```python
from build123d import *

# Parameters (mm, degrees)
SKETCH2_R           = 3.65
BOSS_EXTRUDE1_DEPTH = 1.4
SKETCH3_R           = 2.8
BOSS_EXTRUDE2_DEPTH = 5.2
SKETCH4_R           = 3.65
BOSS_EXTRUDE3_DEPTH = 1.4
CUT_EXTRUDE1_DEPTH  = 9
CUT_EXTRUDE2_DEPTH  = 14.65


with BuildPart() as part:
    # Sketch2 → Boss-Extrude1 (new body)
    with BuildSketch(Plane(origin=(0, 0, 0), x_dir=(1, 0, 0), z_dir=(0, 1, 0))):
        Circle(SKETCH2_R)
    extrude(amount=BOSS_EXTRUDE1_DEPTH)

    # Sketch3 → Boss-Extrude2 (add)
    with BuildSketch(Plane(origin=(0, 1.4, 0), x_dir=(1, 0, 0), z_dir=(0, 1, 0))):
        Circle(SKETCH3_R)
    extrude(amount=BOSS_EXTRUDE2_DEPTH)

    # Sketch4 → Boss-Extrude3 (add)
    with BuildSketch(Plane(origin=(0, 6.6, 0), x_dir=(1, 0, 0), z_dir=(0, 1, 0))):
        Circle(SKETCH4_R)
    extrude(amount=BOSS_EXTRUDE3_DEPTH)

    # Sketch5 → Cut-Extrude1 (cut, through all)
    with BuildSketch(Plane(origin=(0, 8, 0), x_dir=(1, 0, 0), z_dir=(0, 1, 0))):
        Polygon((0.85, -2.351063589), (0.85, -0.85), (2.351063589, -0.85), (2.351063589, 0.85), (0.85, 0.85), (0.85, 2.351063589), (-0.85, 2.351063589), (-0.85, 0.85), (-2.351063589, 0.85), (-2.351063589, -0.85), (-0.85, -0.85), (-0.85, -2.351063589), align=None)
    extrude(amount=-CUT_EXTRUDE1_DEPTH, mode=Mode.SUBTRACT)

    # Sketch6 → Cut-Extrude2 (cut, through all)
    with BuildSketch(Plane(origin=(10, 0, 0), x_dir=(0, 0, -1), z_dir=(1, 0, 0))):
        with BuildLine():
            Line((0.5, 6.098665366), (0.5, 1.901334634))
            ThreePointArc((0.5, 1.901334634), (0, 1.401334634), (-0.5, 1.901334634))
            Line((-0.5, 1.901334634), (-0.5, 6.098665366))
            ThreePointArc((-0.5, 6.098665366), (0, 6.598665366), (0.5, 6.098665366))
        make_face()
    extrude(amount=-CUT_EXTRUDE2_DEPTH, mode=Mode.SUBTRACT)


solid = part.part
```
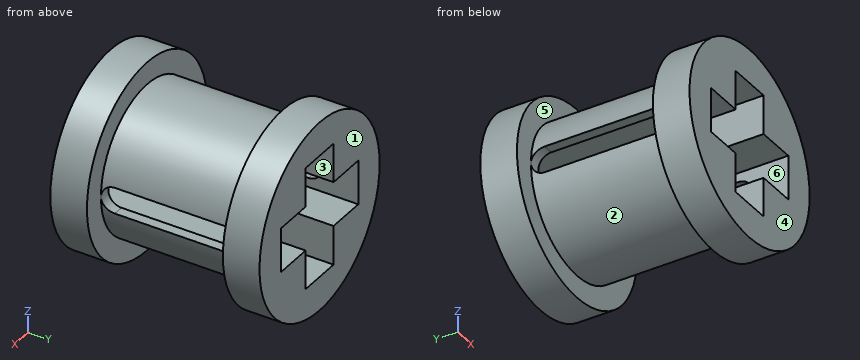
Part model, mm, in its own coordinate system. Face numbers are marked on the shaded views. A direction names the side the tool comes from. Round coordinates to 2 decimals unless told otherwise and drop trailing zeros. Loops run counter-clockwise (first coordinate to the right, second up) from the corner with the lowest first, then second, coordinate; pieces in that order, holes last.
Item 1: Drill centre lines: line 1 (Y direction, x = 0, z = 3); line 2 (X direction, y = 0.75, z = 1.5); line 3 (X direction, y = 2.5, z = -2). Where is each one in solid material? Low to high.
Item 2: Cut at D-D, the plane z = 1. Give the cut face in (x, y), then the cut area to 3 significant figures.
Item 3: Cut at A-A, the plane x = 0. Give the cut face in (y, z), then the cut area to 3 significant figures.
Item 4: Drop flat-ended pins along their axis: P1, Ø1.2, axis at y = 4, z = 2, coming from the +X side; P2, Ø2, axis at y = 6.5, z = 2, coming from the +X side; P3, Ø1.7, axis at x = 2, y = 3, coming from the +Z side. Give the stop position or say it passes through.
Item 5: Cut at B-B, the plane z = 0. State how many separate pieces and enclosed holes the cut face has, then the cut area to 3 significant figures.
Item 6: Mould opens along Z. For the marked faces 1, 2 and 3 say: +Z half, -Z half, draft (parallel to the pull), parting line (faces both ways), or undercut.
Item 7: 3-axis set-ups, long thin cutter, end or side, ignore diameter. For the marked faces 4, 5 and 6: which of +Z, -Z, +X, -X, +Y, -Y reach the whole face in a straight line?
Item 8: Cut at C-C, the plane y = 0.5. Give the cut face in (x, z).
A:
1. line 1: y = 0 to 1.4, 6.6 to 8
1. line 2: x = -3.33 to -0.85, 0.85 to 3.33
1. line 3: x = -1.96 to -0.85, 0.85 to 1.96
2. outline: (-3.51, 0) - (-0.85, 0) - (-0.85, 8) - (-3.51, 8) - (-3.51, 6.6) - (-2.62, 6.6) - (-2.62, 1.4) - (-3.51, 1.4) - close; (0.85, 0) - (3.51, 0) - (3.51, 1.4) - (2.62, 1.4) - (2.62, 6.6) - (3.51, 6.6) - (3.51, 8) - (0.85, 8) - close
2. area: 33.3 mm2
3. outline: (0, -3.65) - (1.4, -3.65) - (1.4, -2.8) - (6.6, -2.8) - (6.6, -3.65) - (8, -3.65) - (8, -2.35) - (0, -2.35) - close; (0, 2.35) - (8, 2.35) - (8, 3.65) - (6.6, 3.65) - (6.6, 2.8) - (1.4, 2.8) - (1.4, 3.65) - (0, 3.65) - close
3. area: 11.9 mm2
4. P1: stops at x = 2.42
4. P2: stops at x = 3.51
4. P3: stops at z = 2.55
5. separate pieces: 4
5. enclosed holes: 0
5. area: 7.28 mm2
6. face 1: draft
6. face 2: parting line
6. face 3: undercut
7. face 4: +Z, -Z, +X, -X, -Y
7. face 5: none
7. face 6: +Y, -Y
8. outline: circle Ø7.3 at (0, 0); hole (-2.35, -0.85) - (-0.85, -0.85) - (-0.85, -2.35) - (0.85, -2.35) - (0.85, -0.85) - (2.35, -0.85) - (2.35, 0.85) - (0.85, 0.85) - (0.85, 2.35) - (-0.85, 2.35) - (-0.85, 0.85) - (-2.35, 0.85) - close
